Can you work these out from the model? Positions are in its coordinate system, mm. Face numbers are marked on the shaded views. Give positions to 0.01 mm unless a question says otherwise; leave off trailing zeros. Loops run counter-clockwise (first coordinate to the right, second up) from the corner with the lowest first, then second, coordinate; pieces in that order, holes last. Notation, with made-up numbers: (-23, 11.5) - (-13, 11.5) arc R25 ccw to (-13, 31.5) - close; hole circle Ø1 at (-33, 72.5). An arc over 180 degrees is marked (long way). Answer in a Markdown table with one row per item.
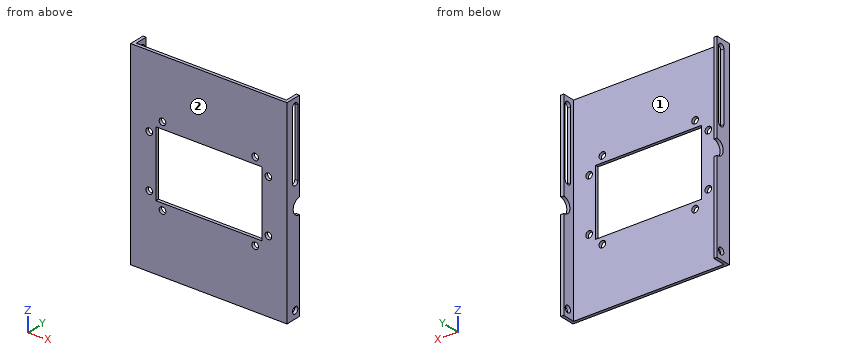
from build123d import *

# Parameters (mm, degrees)
EXTRUDE_THIN1_DEPTH      = 95
EXTRUDE_THIN1_DEPTH_BACK = 95
SKETCH2_R                = 3.2385
CUT_EXTRUDE1_DEPTH       = 179.185296812
CUT_EXTRUDE2_DEPTH       = 179.185296812
CUT_EXTRUDE2_DEPTH_BACK  = 179.185296812
SKETCH3_R                = 7.5
SKETCH4_R                = 3.175
SKETCH4_W                = 101.6
SKETCH4_H                = 63.5
CUT_EXTRUDE3_DEPTH       = 10


with BuildPart() as part:
    # Sketch1 → Extrude-Thin1 (new, two sides: drawn at the far end of the back side and taken through both)
    with BuildSketch(Plane.XY.offset(-EXTRUDE_THIN1_DEPTH_BACK)):
        Polygon((-75, 15), (-75, 0), (75, 0), (75, 15), (72, 15), (72, 3), (-72, 3), (-72, 15), align=None)
    extrude(amount=EXTRUDE_THIN1_DEPTH + EXTRUDE_THIN1_DEPTH_BACK)

    # Sketch2 → Cut-Extrude1 (cut, through all)
    with BuildSketch(Plane.ZY.offset(75)):
        with Locations((-87.5, 10)):
            Circle(SKETCH2_R)
        with BuildLine():
            Line((87.5, 6.7615), (22.5, 6.7615))
            ThreePointArc((22.5, 6.7615), (19.2615, 10), (22.5, 13.2385))
            Line((22.5, 13.2385), (87.5, 13.2385))
            ThreePointArc((87.5, 13.2385), (90.7385, 10), (87.5, 6.7615))
        make_face()
    extrude(amount=-CUT_EXTRUDE1_DEPTH, mode=Mode.SUBTRACT)

    # Sketch3 → Cut-Extrude2 (cut, two sides: drawn at the far end of the back side and taken through both)
    with BuildSketch(Plane(origin=(75, 0, 0), x_dir=(0, 0, -1), z_dir=(1, 0, 0)).offset(-CUT_EXTRUDE2_DEPTH_BACK)):
        with Locations((0, 15)):
            Circle(SKETCH3_R)
    extrude(amount=CUT_EXTRUDE2_DEPTH + CUT_EXTRUDE2_DEPTH_BACK, mode=Mode.SUBTRACT)

    # Sketch4 → Cut-Extrude3 (cut)
    with BuildSketch(Plane(origin=(0, 3, 0), x_dir=(1, 0, 0), z_dir=(0, 1, 0))):
        with Locations(Location((-44.45, 38.1, 0), (0, 0, 270))):
            Circle(SKETCH4_R)
        with Locations(Location((44.45, 38.1, 0), (0, 0, 270))):
            Circle(SKETCH4_R)
        with Locations(Location((-44.45, -38.1, 0), (0, 0, 270))):
            Circle(SKETCH4_R)
        with Locations(Location((44.45, -38.1, 0), (0, 0, 270))):
            Circle(SKETCH4_R)
        with Locations(Location((-57.15, 25.4, 0), (0, 0, 270))):
            Circle(SKETCH4_R)
        with Locations(Location((57.15, 25.4, 0), (0, 0, 270))):
            Circle(SKETCH4_R)
        with Locations(Location((-57.15, -25.4, 0), (0, 0, 270))):
            Circle(SKETCH4_R)
        with Locations(Location((57.15, -25.4, 0), (0, 0, 270))):
            Circle(SKETCH4_R)
        Rectangle(SKETCH4_W, SKETCH4_H)
    extrude(amount=-CUT_EXTRUDE3_DEPTH, mode=Mode.SUBTRACT)


solid = part.part
Q1. If we mould it in two halves opening along X, with no side actions, what happens to the marked faces 1 and 2? For each: released by +X, released by -X, zero draft, split by the parting line, or undercut.
Checked values:
| item | result |
|---|---|
| face 1 | undercut |
| face 2 | zero draft |
Q2. Imagine slicing it at B-B, the plane z = 25.4. Write out the boundary of the cut face in (x, y) (1 decimal), and give its area (3 significant figures).
Checked values:
| item | result |
|---|---|
| outline | (-75, 0) - (-60.3, 0) - (-60.3, 3) - (-72, 3) - (-72, 6.8) - (-75, 6.8) - close; (-75, 13.2) - (-72, 13.2) - (-72, 15) - (-75, 15) - close; (-54, 0) - (-50.8, 0) - (-50.8, 3) - (-54, 3) - close; (50.8, 0) - (54, 0) - (54, 3) - (50.8, 3) - close; (60.3, 0) - (75, 0) - (75, 6.8) - (72, 6.8) - (72, 3) - (60.3, 3) - close; (72, 13.2) - (75, 13.2) - (75, 15) - (72, 15) - close |
| area | 140 mm² |
Q3. For pin 1 (5.5 mm diameter, centred on x = -57.15, z = 25.4, fed in from +Y); pin 2 (10 mm diameter, centred on x = 57.15, z = -25.4, fed in from +Y), each with a flat end and sliding along its axis, tell me the tip position at first contact or that it passes through.
Checked values:
| item | result |
|---|---|
| pin 1 | passes through |
| pin 2 | stops at y = 3 |
Q4. If I drill on line 1 (X direction, y = 1, z = 25.4) (3 decimals); line 2 (X direction, y = 0.7, z = 38.1) (3 decimals); line 3 (X direction, y = 4.5, z = 45), over which ranges is the centre line in solid material (lowest first)? Write a range as [from, to].
Checked values:
| item | result |
|---|---|
| line 1 | x = [-75, -60.325], [-53.975, -50.8], [50.8, 53.975], [60.325, 75] |
| line 2 | x = [-75, -47.625], [-41.275, 41.275], [47.625, 75] |
| line 3 | x = [-75, -72], [72, 75] |
Q5. Imagine slicing it at C-C, the plane z = -25.4. Write out the boundary of the cut face in (x, y) (3 decimals).
Checked values:
| item | result |
|---|---|
| outline | (-75, 0) - (-60.325, 0) - (-60.325, 3) - (-72, 3) - (-72, 15) - (-75, 15) - close; (-53.975, 0) - (-50.8, 0) - (-50.8, 3) - (-53.975, 3) - close; (50.8, 0) - (53.975, 0) - (53.975, 3) - (50.8, 3) - close; (60.325, 0) - (75, 0) - (75, 15) - (72, 15) - (72, 3) - (60.325, 3) - close |
Q6. Imagine slicing it at A-A, the plane x = 57.15. Write out the boundary of the cut face in (y, z) (3 decimals).
Checked values:
| item | result |
|---|---|
| outline | (0, -95) - (3, -95) - (3, -28.575) - (0, -28.575) - close; (0, -22.225) - (3, -22.225) - (3, 22.225) - (0, 22.225) - close; (0, 28.575) - (3, 28.575) - (3, 95) - (0, 95) - close |
Q7. Imagine slicing it at D-D, the plane x = -44.45. Write out the boundary of the cut face in (y, z) (3 decimals).
Checked values:
| item | result |
|---|---|
| outline | (0, -95) - (3, -95) - (3, -41.275) - (0, -41.275) - close; (0, -34.925) - (3, -34.925) - (3, -31.75) - (0, -31.75) - close; (0, 31.75) - (3, 31.75) - (3, 34.925) - (0, 34.925) - close; (0, 41.275) - (3, 41.275) - (3, 95) - (0, 95) - close |
